```python
from build123d import *

# Parameters (mm, degrees)
F0_W     = 20
F0_H     = 20
F1_DEPTH = 20
F3_W     = 17
F3_H     = 17
F4_DEPTH = 30
F5_W     = 17
F5_H     = 17
F6_DEPTH = 30


with BuildPart() as f1:
    # F0 (on Front) → F1 (new body)
    with BuildSketch(Plane.XZ):
        Rectangle(F0_W, F0_H)
    extrude(amount=F1_DEPTH)


with BuildPart() as f1_1:
    # F2: moved
    add(f1.part.moved(Location((0, 10, 0))))

    # F3 (on face) → F4 (join)
    with BuildSketch(Plane.XZ.offset(10)):
        Rectangle(F3_W, F3_H)
    extrude(amount=F4_DEPTH)

    # F5 (on face) → F6 (join)
    with BuildSketch(Plane.YZ.offset(10)):
        Rectangle(F5_W, F5_H)
    extrude(amount=F6_DEPTH)


solid = f1_1.part
```
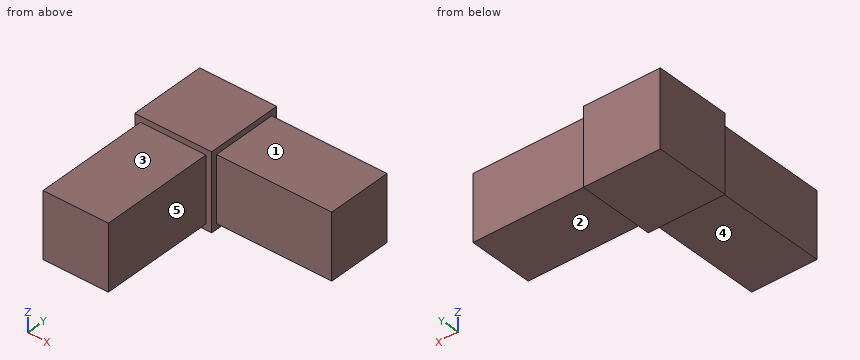
Build history of the part. All positions in model axes, mm. Face numbers are marked on the shaded views. A direction names the side the tool comes from. Round coordinates to 2 decimals unless told otherwise and drop trailing zeros. Loops run counter-clockwise (first coordinate to the right, second up) from the corner with the lowest first, then second, coordinate; pieces in that order, holes last.
Item 1: Saw through at D-D (y = -31.5). List the corners of the cut face in (x, z), then the cut area to 3 significant figures.
Item 2: Saw through at C-C (x = 6.5). List the corners of the cut face in (y, z).
Item 3: Saw through at A-A (y = -4.5). List the corners of the cut face in (x, z), then the cut area to 3 significant figures.
Item 4: Which spindle directions (+Z, -Z, +X, -X, +Y, -Y) get a long thin tool onto all of the face, cutting with end or side? Do the marked faces 1, 2, 3, 4 and 5. Say none if no direction does.
Item 5: Drill centre line: line 1 along Z through (x, y) = (34.5, -3). Where is it in solid material? Low to high.
Item 6: Pin check, flat tips, straight feed: P1, Ø8.5, axis at x = -4, y = -22, coming from the +Z side; P2, Ø10, axis at y = -24.5, z = 0.5, coming from the +X side; P3, Ø18.5, axis at x = 29.5, y = -2.5, coming from the -Z side. Stop position of each tip, or through.
Item 7: Saw through at B-B (z = 2). List the corners of the cut face in (x, y).
Worked answers:
1. outline: (-8.5, -8.5) - (8.5, -8.5) - (8.5, 8.5) - (-8.5, 8.5) - close
1. area: 289 mm2
2. outline: (-40, -8.5) - (-10, -8.5) - (-10, -10) - (10, -10) - (10, 10) - (-10, 10) - (-10, 8.5) - (-40, 8.5) - close
3. outline: (-10, -10) - (10, -10) - (10, -8.5) - (40, -8.5) - (40, 8.5) - (10, 8.5) - (10, 10) - (-10, 10) - close
3. area: 910 mm2
4. face 1: +Z, +X, +Y, -Y
4. face 2: -Z, +X, +Y, -Y
4. face 3: +Z, +X, -X, -Y
4. face 4: -Z, +X, -X, -Y
4. face 5: +Z, -Z, +X, -Y
5. line 1: z = -8.5 to 8.5
6. P1: stops at z = 8.5
6. P2: stops at x = 8.5
6. P3: stops at z = -8.5
7. outline: (-10, -10) - (-8.5, -10) - (-8.5, -40) - (8.5, -40) - (8.5, -10) - (10, -10) - (10, -8.5) - (40, -8.5) - (40, 8.5) - (10, 8.5) - (10, 10) - (-10, 10) - close
